Geometry check sheet. Reference: drawing and pictorial views, mm from the part's lowest x, y, z. A direction names the side the tool comes from. Round coordinates to 2 decimals unless told otherwise and drop trailing zeros. Loops run counter-clockwise (first coordinate to the right, second up) from the corner with the lowest first, then second, coordinate; pieces in that order, holes last. Notation, with made-up numbers: (39, -29) -> (47, -29) arc R28 ccw to (47, -10) -> close; hole circle Ø6 at (37.5, 89). An arc over 180 degrees is marked (long way). Write item = value, one per line.
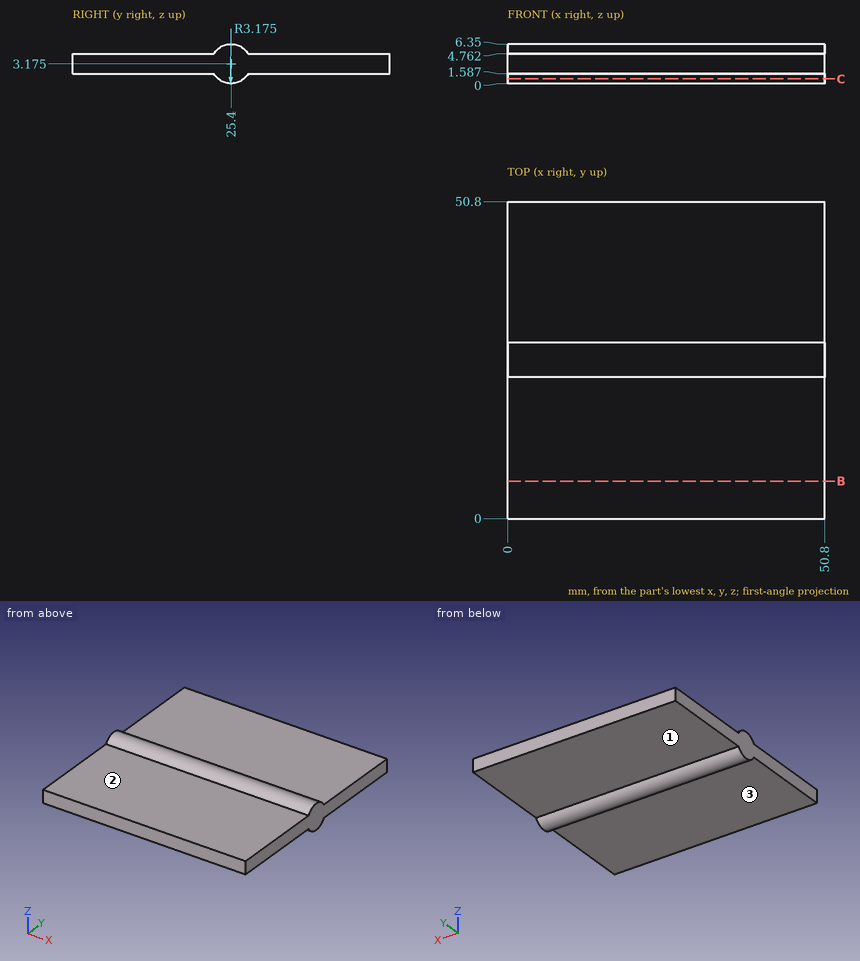
(1) Sectioned sample at C-C, the plane z = 0.75. Record the cut outline in (x, y), and give its area (3 significant figures).
Filled sheet:
outline = (0, 23.35) -> (50.8, 23.35) -> (50.8, 27.45) -> (0, 27.45) -> close
area = 208 mm2
(2) Material ranges on probe 1 along Z at (x, y) = (41, 46.5); probe 2 along Z at (x, y) = (8, 25.5); probe 3 along Y at (x, z) = (46.5, 5.75) (1 decimal), recorded low to high. Write a range as from..to.
Filled sheet:
probe_1 = 1.59..4.76
probe_2 = 0..6.35
probe_3 = 23.5..27.3
(3) Sectioned sample at B-B, the plane y = 6. Record the cut outline in (x, z).
Filled sheet:
outline = (0, 1.59) -> (50.8, 1.59) -> (50.8, 4.76) -> (0, 4.76) -> close
(4) Set-up check for the marked faces 1, 2 and 3: record each of +Z, -Z, +X, -X, +Y, -Y from which the full face is reachable in a straight line by a thin tool's end or side.
Filled sheet:
face_1 = -Z, +X, -X, +Y
face_2 = +Z, +X, -X, -Y
face_3 = -Z, +X, -X, -Y
(5) Go/stop test with flat-tipped pins: pin 1 Ø7 at (x, y) = (24, 14.5) entering from -Z; pin 2 Ø11.5 at (x, y) = (26, 8.5) entering from +Z. Record where each tip stops, or that it passes through.
Filled sheet:
pin_1 = 1.59
pin_2 = 4.76
